from build123d import *

# Parameters (mm, degrees)
SKETCH1_W               = 203.2
SKETCH1_H               = 146.05
BOSS_EXTRUDE1_DEPTH     = 6.35
CUT_EXTRUDE1_DEPTH      = 251.322122474
CUT_EXTRUDE1_DEPTH_BACK = 251.322122474
SKETCH2_R               = 3.175
CUT_EXTRUDE2_DEPTH      = 251.322122474
CUT_EXTRUDE2_DEPTH_BACK = 251.322122474
SKETCH3_R               = 2.032
CUT_EXTRUDE3_DEPTH      = 251.322122474
CUT_EXTRUDE3_DEPTH_BACK = 251.322122474
SKETCH4_W               = 57.15
SKETCH4_H               = 66.675
FILLET1_R               = 12.7


with BuildPart() as part:
    # Sketch1 → Boss-Extrude1 (new body)
    with BuildSketch(Plane.XY):
        with Locations((101.6, 73.025)):
            Rectangle(SKETCH1_W, SKETCH1_H)
    extrude(amount=BOSS_EXTRUDE1_DEPTH)

    # Sketch2 → Cut-Extrude1 (cut, two sides: drawn at the far end of the back side and taken through both)
    with BuildSketch(Plane.XY.offset(6.35).offset(-CUT_EXTRUDE1_DEPTH_BACK)):
        with Locations((12.7, 6.35)):
            Circle(SKETCH2_R)
        with Locations((38.1, 6.35)):
            Circle(SKETCH2_R)
        with Locations((12.7, 95.25)):
            Circle(SKETCH2_R)
        with Locations((38.1, 95.25)):
            Circle(SKETCH2_R)
        with Locations((190.5, 95.25)):
            Circle(SKETCH2_R)
        with Locations((190.5, 6.35)):
            Circle(SKETCH2_R)
        with Locations((12.7, 69.85)):
            Circle(SKETCH2_R)
        with Locations((38.1, 69.85)):
            Circle(SKETCH2_R)
        with Locations((12.7, 44.45)):
            Circle(SKETCH2_R)
        with Locations((38.1, 44.45)):
            Circle(SKETCH2_R)
        with Locations((12.7, 120.65)):
            Circle(SKETCH2_R)
        with Locations((38.1, 120.65)):
            Circle(SKETCH2_R)
        with Locations((165.1, 6.35)):
            Circle(SKETCH2_R)
        with Locations((139.7, 6.35)):
            Circle(SKETCH2_R)
    extrude(amount=CUT_EXTRUDE1_DEPTH + CUT_EXTRUDE1_DEPTH_BACK, mode=Mode.SUBTRACT)

    # Sketch3 → Cut-Extrude2 (cut, two sides: drawn at the far end of the back side and taken through both)
    with BuildSketch(Plane.XY.offset(6.35).offset(-CUT_EXTRUDE2_DEPTH_BACK)):
        with Locations((95.25, 139.7)):
            Circle(SKETCH3_R)
        with Locations((107.95, 139.7)):
            Circle(SKETCH3_R)
        with Locations((82.55, 139.7)):
            Circle(SKETCH3_R)
        with Locations((107.95, 127)):
            Circle(SKETCH3_R)
        with Locations((95.25, 127)):
            Circle(SKETCH3_R)
        with Locations((82.55, 127)):
            Circle(SKETCH3_R)
        with Locations((107.95, 114.3)):
            Circle(SKETCH3_R)
        with Locations((95.25, 114.3)):
            Circle(SKETCH3_R)
        with Locations((82.55, 114.3)):
            Circle(SKETCH3_R)
        with Locations((107.95, 101.6)):
            Circle(SKETCH3_R)
        with Locations((95.25, 101.6)):
            Circle(SKETCH3_R)
        with Locations((82.55, 101.6)):
            Circle(SKETCH3_R)
        with Locations((107.95, 88.9)):
            Circle(SKETCH3_R)
        with Locations((95.25, 88.9)):
            Circle(SKETCH3_R)
        with Locations((82.55, 88.9)):
            Circle(SKETCH3_R)
    extrude(amount=CUT_EXTRUDE2_DEPTH + CUT_EXTRUDE2_DEPTH_BACK, mode=Mode.SUBTRACT)

    # Sketch4 → Cut-Extrude3 (cut, two sides: drawn at the far end of the back side and taken through both)
    with BuildSketch(Plane.XY.offset(6.35).offset(-CUT_EXTRUDE3_DEPTH_BACK)):
        with Locations((95.25, 49.2125)):
            Rectangle(SKETCH4_W, SKETCH4_H)
    extrude(amount=CUT_EXTRUDE3_DEPTH + CUT_EXTRUDE3_DEPTH_BACK, mode=Mode.SUBTRACT)

    # Fillet1
    fillet1_edges = [part.edges().sort_by_distance(p)[0] for p in [
        (66.675, 15.875, 3.175),
        (66.675, 82.55, 3.175),
        (123.825, 82.55, 3.175),
        (123.825, 15.875, 3.175),
    ]]
    fillet(fillet1_edges, radius=FILLET1_R)


solid = part.part
Geometry: final body of the model. Coordinates: model frame, mm. A direction names the side the tool comes from. Give positions to 0.01 mm unless a question says otherwise; leave off trailing zeros. Loops run counter-clockwise (first coordinate to the right, second up) from the corner with the lowest first, then second, coordinate; pieces in that order, holes last. Notation, with made-up numbers: (38.25, 11.25) - (65.25, 11.25) arc R24 cw to (65.25, 27.25) - close; hole circle Ø8 at (8.5, 60.5). An arc over 180 degrees is marked (long way). Answer as CSV lines item,"result". Start each with the question number.
1. Pin query (flat end, axial travel): P1, Ø1.5, axis at y = 128.5, z = 1, coming from the -X side; P2, Ø3.5, axis at x = 107.95, y = 139.7, coming from the -Z side. Return the tip coordinate at first contact, or that it passes through.
2. Ray query, L1, parallel to X at y = 95.25, z = 3.25 (3 decimals); L2, parallel to X at y = 101.6, z = 3.5; L3, parallel to Y at x = 190.5, z = 3 (3 decimals). Return the intervals inside material, ascending.
3. Reachability of faces 4 (the face through (100, 90, 6.35)), 5 (the face through (120.01, 19.5, 3.22)) from +Z, -Z, +X, -X, +Y, -Y: full face, straight path, thin tool, end or side. Return the list, or none.
4. Draft query along Y for faces 1 (the face through (100, 0, 3)), 2 (the face through (83.642, 141.413, 3.131)), 3 (the face through (100, 146.05, 3)). Return one class per face: released by +Y, released by -Y, zero draft, split by the parting line, or undercut.
5. Section D-D, the plane x = 82.55. Return loops of the section in (y, z) (3 decimals), plus the area to 3 significant figures.
6. Section C-C, the plane y = 120.65. Return loops of the section in (x, z) (3 decimals).
7. Section B-B, the plane y = 95.25. Return loops of the section in (x, z) (3 decimals).
8. Section A-A, the plane x = 38.1. Return loops of the section in (y, z) (3 decimals), plus the area to 3 significant figures.
Answers:
1,P1,"stops at x = 0"
1,P2,"passes through"
2,L1,"x = 0 to 9.525, 15.875 to 34.925, 41.275 to 187.325, 193.675 to 203.2"
2,L2,"x = 0 to 80.52, 84.58 to 93.22, 97.28 to 105.92, 109.98 to 203.2"
2,L3,"y = 0 to 3.175, 9.525 to 92.075, 98.425 to 146.05"
3,face 4,"+Z, +X, -X, +Y, -Y"
3,face 5,"+Z, -Z"
4,face 1,"released by -Y"
4,face 2,"undercut"
4,face 3,"released by +Y"
5,outline,"(0, 0) - (15.875, 0) - (15.875, 6.35) - (0, 6.35) - close; (82.55, 0) - (86.868, 0) - (86.868, 6.35) - (82.55, 6.35) - close; (90.932, 0) - (99.568, 0) - (99.568, 6.35) - (90.932, 6.35) - close; (103.632, 0) - (112.268, 0) - (112.268, 6.35) - (103.632, 6.35) - close; (116.332, 0) - (124.968, 0) - (124.968, 6.35) - (116.332, 6.35) - close; (129.032, 0) - (137.668, 0) - (137.668, 6.35) - (129.032, 6.35) - close; (141.732, 0) - (146.05, 0) - (146.05, 6.35) - (141.732, 6.35) - close"
5,area,"375 mm2"
6,outline,"(0, 0) - (9.525, 0) - (9.525, 6.35) - (0, 6.35) - close; (15.875, 0) - (34.925, 0) - (34.925, 6.35) - (15.875, 6.35) - close; (41.275, 0) - (203.2, 0) - (203.2, 6.35) - (41.275, 6.35) - close"
7,outline,"(0, 0) - (9.525, 0) - (9.525, 6.35) - (0, 6.35) - close; (15.875, 0) - (34.925, 0) - (34.925, 6.35) - (15.875, 6.35) - close; (41.275, 0) - (187.325, 0) - (187.325, 6.35) - (41.275, 6.35) - close; (193.675, 0) - (203.2, 0) - (203.2, 6.35) - (193.675, 6.35) - close"
8,outline,"(0, 0) - (3.175, 0) - (3.175, 6.35) - (0, 6.35) - close; (9.525, 0) - (41.275, 0) - (41.275, 6.35) - (9.525, 6.35) - close; (47.625, 0) - (66.675, 0) - (66.675, 6.35) - (47.625, 6.35) - close; (73.025, 0) - (92.075, 0) - (92.075, 6.35) - (73.025, 6.35) - close; (98.425, 0) - (117.475, 0) - (117.475, 6.35) - (98.425, 6.35) - close; (123.825, 0) - (146.05, 0) - (146.05, 6.35) - (123.825, 6.35) - close"
8,area,"726 mm2"
